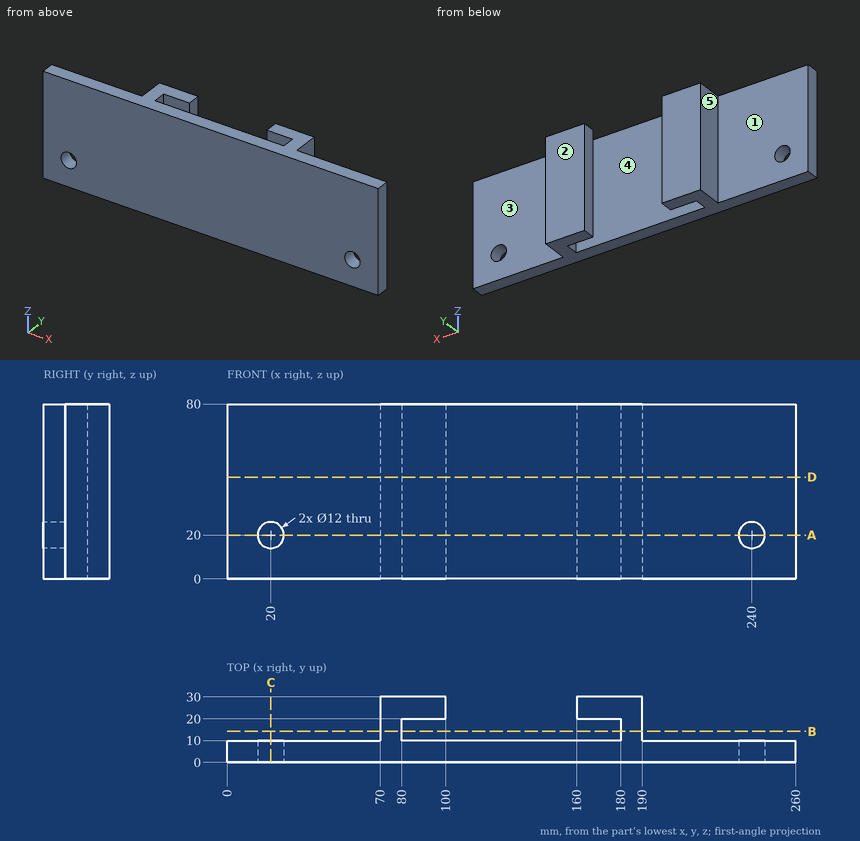
Study the drawing (mm; zero at the part's minimum x, y, z) and answer. A direction names the side the tool comes from. Round coordinates to 2 decimals unless told otherwise and drop trailing zeros. Write each loop counter-clockwise with the first axis right and the second up, starting at its lowest first coordinate (ties: lowest second). Pieces come first, ordered by that corner, then holes.
1) Consider probe 1 along X at (y, z) = (5, 20); probe 2 along X at (y, z) = (14.5, 74.5); probe 3 along X at (y, z) = (25.5, 30). Determine where each line is inside the solid, lowest interval first.
2) A cutting plane is placed at C-C on x = 20. Determine the outline of the cut face in (y, z).
3) Determine the mould class of the marked faces 3, 4 and 5 for opening direction X: pulls with the +X half, pulls with the -X half, needs draft (parallel to the pull), parting line crosses it, or undercut.
4) Flat-ended cylindrical pins translate along their axes: P1, Ø12, axis at y = 18.5, z = 29, coming from the -X side; P2, Ø10, axis at y = 22, z = 8.5, coming from the +X side; P3, Ø2, axis at x = 223.5, y = 12.5, coming from the -Z side; P4, Ø1.5, axis at x = 52, z = 53, coming from the +Y side. Find the tip coordinate at first contact, or state that the pin passes through.
5) A cutting plane is placed at A-A on z = 20. Determine the outline of the cut face in (x, y), and give its area (3 significant figures).
6) A cutting plane is placed at D-D on z = 46.5. Determine the outline of the cut face in (x, y), and give its area (3 significant figures).
7) Which of the six approach directions +Z, -Z, +X, -X, +Y, -Y give full straight-line access (tool end or side, diameter ignored) to the marked faces 1 and 2?
8) A cutting plane is placed at B-B on y = 14.25. Determine the outline of the cut face in (x, z), and give its area (3 significant figures).
Entries:
1. probe 1: x = 0 to 14, 26 to 234, 246 to 260
1. probe 2: x = 70 to 80, 180 to 190
1. probe 3: x = 70 to 100, 160 to 190
2. outline: (0, 0) - (10, 0) - (10, 14) - (0, 14) - close; (0, 26) - (10, 26) - (10, 80) - (0, 80) - close
3. face 3: needs draft
3. face 4: undercut
3. face 5: pulls with the -X half
4. P1: stops at x = 70
4. P2: stops at x = 190
4. P3: passes through
4. P4: stops at y = 10
5. outline: (0, 0) - (14, 0) - (14, 10) - (0, 10) - close; (26, 0) - (234, 0) - (234, 10) - (190, 10) - (190, 30) - (160, 30) - (160, 20) - (180, 20) - (180, 10) - (80, 10) - (80, 20) - (100, 20) - (100, 30) - (70, 30) - (70, 10) - (26, 10) - close; (246, 0) - (260, 0) - (260, 10) - (246, 10) - close
5. area: 3,160 mm2
6. outline: (0, 0) - (260, 0) - (260, 10) - (190, 10) - (190, 30) - (160, 30) - (160, 20) - (180, 20) - (180, 10) - (80, 10) - (80, 20) - (100, 20) - (100, 30) - (70, 30) - (70, 10) - (0, 10) - close
6. area: 3,400 mm2
7. face 1: +Z, -Z, -X, +Y
7. face 2: +Z, -Z, +X, -X, +Y
8. outline: (70, 0) - (80, 0) - (80, 80) - (70, 80) - close; (180, 0) - (190, 0) - (190, 80) - (180, 80) - close
8. area: 1,600 mm2
